Design review of the part built by this model. Coordinates are the model's own, in mm. A direction names the side the tool comes from. Coordinates: 2 decimals unless noted, no trailing zeros. Loops run counter-clockwise (first coordinate to the right, second up) from the corner with the lowest first, then second, coordinate; pieces in that order, holes last. Notation, with made-up numbers: M 37,-13.75 L 78,-13.75 A20 cw 78,21.25 Z; hole C -21.5,74.25 d1. An arc over 180 degrees is marked long. Write item = value, one per line. Start each with the question number.
```python
from build123d import *

# Parameters (mm, degrees)
F0_W     = 119.359527
F0_H     = 100.470527
F1_DEPTH = 72.39
F2_R     = 25.4
F3_R     = 25.4
F4_R     = 25.4
F5_R     = 25.4
F6_T     = -2.54


with BuildPart() as f1:
    # F0 (on Front) → F1 (new body)
    with BuildSketch(Plane.XZ):
        with Locations((-9.005385, 12.515958)):
            Rectangle(F0_W, F0_H)
    extrude(amount=F1_DEPTH)

    # F2
    f2_edges = [f1.edges().sort_by_distance(p)[0] for p in [
        (-9.005385, -72.39, 62.751222),
    ]]
    fillet(f2_edges, radius=F2_R)

    # F3
    f3_edges = [f1.edges().sort_by_distance(p)[0] for p in [
        (-9.005385, 0, 62.751222),
    ]]
    fillet(f3_edges, radius=F3_R)

    # F4
    f4_edges = [f1.edges().sort_by_distance(p)[0] for p in [
        (50.674379, -36.195, 62.751222),
    ]]
    fillet(f4_edges, radius=F4_R)

    # F5
    f5_edges = [f1.edges().sort_by_distance(p)[0] for p in [
        (-68.685148, -36.195, 62.751222),
    ]]
    fillet(f5_edges, radius=F5_R)

    # F6
    f6_openings = [f1.faces().sort_by_distance(p)[0] for p in [
        (-9.005385, -36.195, -37.719305),
    ]]
    offset(amount=F6_T, openings=f6_openings)


solid = f1.part
```
(1) Take a section at D-D (z = 40.5). State the section outline as (x, y) points, plus the area to 3 significant figures.
(2) Insertion check: pin 1 (17.5 mm diameter, centred on x = -15.5, y = -31.5, fed in from -Z); pin 2 (12 mm diameter, centred on y = -22, z = -4.5, fed in from +X); pin 3 (5 mm diameter, centred on x = 27.5, y = -60.5, fed in from -Z); pin 4 (1 mm diameter, centred on x = 30, z = 33.5, fed in from -Y). Each pin has a flat end and moves straight along its axis. Give the tip position at first contact, or say it passes through.
(3) Take a section at B-B (y = -43). State the section outline as (x, z) points.
(4) To check wall thickness, follow L1, parallel to X at y = -35.5, z = -10; L2, parallel to Y at x = -31, z = 7; L3, parallel to Y at x = -44.5, z = 24.5. State the ranges of each line that lie inside material, in increasing order.
(5) Mouldability with a two-part tool opening along X and no side actions: class faces 1 (the flat face through (-9, -72.39, 0)), 2 (the cylindrical face through (43.036, -7.243, 0.341)), 3 (the cylindrical face through (41.26, -63.33, -0.71)), 4 (the flat face through (-68.685, -36, -1)) as +X half, -X half, draft (parallel to the pull), parting line (faces both ways), or undercut.
(6) Take a section at C-C (x = 22.5). State the section outline as (y, z) points, plus the area to 3 significant figures.
(7) Tool access review of faces 5 (the flat face through (-9, -2.54, 0)), 6 (the flat face through (-9, -36, 62.751)): name each direction out of +Z, -Z, +X, -X, +Y, -Y from which nothing blocks a thin tool from reaching the whole face with its end or side.
(8) Take a section at A-A (z = -27.5). State the section outline as (x, y) points, plus the area to 3 significant figures.
Results list:
q1.outline = M -68.49,-46.99 A25.2 ccw -43.29,-72.19 L 25.27,-72.19 A25.2 ccw 50.48,-46.99 L 50.48,-25.4 A25.2 ccw 25.27,-0.2 L -43.29,-0.2 A25.2 ccw -68.49,-25.4 Z; hole M -65.93,-46.99 A22.64 ccw -43.29,-69.63 L 25.27,-69.63 A22.64 ccw 47.92,-46.99 L 47.92,-25.4 A22.64 ccw 25.27,-2.76 L -43.29,-2.76 A22.64 ccw -65.93,-25.4 Z
q1.area = 847 mm^2
q2.pin_1 = 60.06
q2.pin_2 = 50.67
q2.pin_3 = 53.49
q2.pin_4 = -72.04
q3.outline = M -68.69,-37.72 L -66.15,-37.72 L -66.15,37.35 A22.86 cw -43.29,60.21 L 25.27,60.21 A22.86 cw 48.13,37.35 L 48.13,-37.72 L 50.67,-37.72 L 50.67,37.35 A25.4 ccw 25.27,62.75 L -43.29,62.75 A25.4 ccw -68.69,37.35 Z
q4.L1 = -68.69 to -66.15, 48.13 to 50.67
q4.L2 = -72.39 to -69.85, -2.54 to 0
q4.L3 = -72.36 to -69.82, -2.57 to -0.03
q5.face_1 = draft
q5.face_2 = +X half
q5.face_3 = undercut
q5.face_4 = -X half
q6.outline = M -72.39,-37.72 L -69.85,-37.72 L -69.85,37.35 A22.86 cw -46.99,60.21 L -25.4,60.21 A22.86 cw -2.54,37.35 L -2.54,-37.72 L 0,-37.72 L 0,37.35 A25.4 ccw -25.4,62.75 L -46.99,62.75 A25.4 ccw -72.39,37.35 Z
q6.area = 629 mm^2
q7.face_5 = -Z
q7.face_6 = +Z, +X, -X, +Y, -Y
q8.outline = M -68.69,-46.99 A25.4 ccw -43.29,-72.39 L 25.27,-72.39 A25.4 ccw 50.67,-46.99 L 50.67,-25.4 A25.4 ccw 25.27,0 L -43.29,0 A25.4 ccw -68.69,-25.4 Z; hole M -66.15,-46.99 A22.86 ccw -43.29,-69.85 L 25.27,-69.85 A22.86 ccw 48.13,-46.99 L 48.13,-25.4 A22.86 ccw 25.27,-2.54 L -43.29,-2.54 A22.86 ccw -66.15,-25.4 Z
q8.area = 843 mm^2
